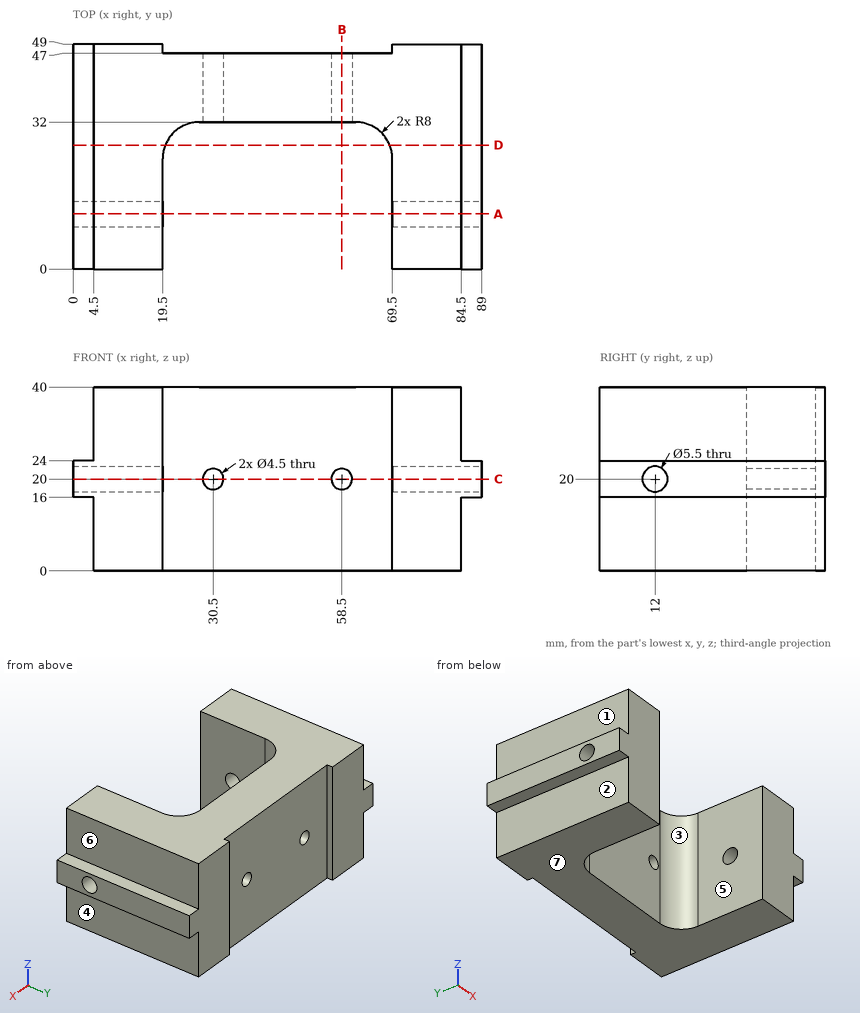
Geometry check sheet. Reference: drawing and pictorial views, mm from the part's lowest x, y, z. A direction names the side the tool comes from. Coordinates: 2 decimals unless noted, no trailing zeros. Write each loop counter-clockwise with the first axis right and the second up, starting at its lowest first coordinate (ties: lowest second). Pieces come first, ordered by that corner, then holes. Notation, with made-up numbers: (-26, -37.75) - (6, -37.75) arc R15 ccw to (6, -19.75) - close; hole circle Ø7 at (37, 78.25). An arc over 180 degrees is marked (long way). One line per question, with ' | ' between items. Start each with the question number.
1. Gauge pin test, flat ends, axial feed: P1, Ø2, axis at x = 1.5, y = 22.5, coming from the -Z side; P2, Ø5, axis at y = 16, z = 28.5, coming from the -X side; P3, Ø5, axis at y = 12, z = 20, coming from the +X side; P4, Ø3.5, axis at x = 87, y = 27, coming from the +Z side. Record the tip position at first contact, or that the pin passes through.
2. Section check B-B (x = 58.5). Enter the section's corners in (y, z).
3. Material ranges on line 1 along X through (y, z) = (41.5, 20); line 2 along X through (y, z) = (22.5, 34.5); line 3 along X through (y, z) = (21.5, 18), recorded low to high.
4. Draft check along X on the marked faces 5, 6 and 7. Enter one of: released by +X, released by -X, zero draft, split by the parting line, or undercut.
5. Section check D-D (y = 27). Enter the section's corners in (x, z), plus the area to 3 significant figures.
6. Section check A-A (y = 12). Enter the section's corners in (x, z).
7. Section check C-C (z = 20). Count the separate pieces of the cut face and the enclosed holes in it, plus the area to 3 significant figures.
8. Access from +Z, -Z, +X, -X, +Y, -Y to the whole of each face (thin tool, end or side, straight path). Record for the marked faces 1, 2, 3 and 4.
Computed values:
1) P1: z = 16 | P2: x = 4.5 | P3: through | P4: z = 24
2) outline: (32, 0) - (47, 0) - (47, 17.75) - (32, 17.75) - close; (32, 22.25) - (47, 22.25) - (47, 40) - (32, 40) - close
3) line 1: 0 to 28.25, 32.75 to 56.25, 60.75 to 89 | line 2: 4.5 to 19.5, 69.5 to 84.5 | line 3: 0 to 19.5, 69.5 to 89
4) face 5: undercut | face 6: released by +X | face 7: zero draft
5) outline: (0, 16) - (4.5, 16) - (4.5, 0) - (20.08, 0) - (20.08, 40) - (4.5, 40) - (4.5, 24) - (0, 24) - close; (68.92, 0) - (84.5, 0) - (84.5, 16) - (89, 16) - (89, 24) - (84.5, 24) - (84.5, 40) - (68.92, 40) - close | area: 1,320 mm²
6) outline: (0, 16) - (4.5, 16) - (4.5, 0) - (19.5, 0) - (19.5, 17.25) - (0, 17.25) - close; (0, 22.75) - (19.5, 22.75) - (19.5, 40) - (4.5, 40) - (4.5, 24) - (0, 24) - close; (69.5, 0) - (84.5, 0) - (84.5, 16) - (89, 16) - (89, 17.25) - (69.5, 17.25) - close; (69.5, 22.75) - (89, 22.75) - (89, 24) - (84.5, 24) - (84.5, 40) - (69.5, 40) - close
7) separate pieces: 5 | enclosed holes: 0 | area: 2,340 mm²
8) face 1: +Z, -X, +Y, -Y | face 2: -Z, -X, +Y, -Y | face 3: +Z, -Z, -Y | face 4: -Z, +X, +Y, -Y
